Source: CAD feature listing. Evaluate the final solid. Frame: model axes, mm. A direction names the side the tool comes from. Coordinates: 2 decimals unless noted, no trailing zeros. Loops run counter-clockwise (first coordinate to the right, second up) from the corner with the lowest first, then second, coordinate; pieces in that order, holes last.
from build123d import *

# Parameters (mm, degrees)
SKETCH1_W           = 32
SKETCH1_H           = 32
BOSS_EXTRUDE1_DEPTH = 10
SKETCH2_R           = 11
CUT_EXTRUDE1_DEPTH  = 7
SKETCH3_R           = 2
SKETCH3_R_2         = 7.5
CUT_EXTRUDE2_DEPTH  = 11


with BuildPart() as part:
    # Sketch1 → Boss-Extrude1 (new body)
    with BuildSketch(Plane(origin=(0, 0, 0), x_dir=(1, 0, 0), z_dir=(0, 1, 0))):
        Rectangle(SKETCH1_W, SKETCH1_H)
    extrude(amount=BOSS_EXTRUDE1_DEPTH)

    # Sketch2 → Cut-Extrude1 (cut)
    with BuildSketch(Plane(origin=(0, 10, 0), x_dir=(1, 0, 0), z_dir=(0, 1, 0))):
        Circle(SKETCH2_R)
    extrude(amount=-CUT_EXTRUDE1_DEPTH, mode=Mode.SUBTRACT)

    # Sketch3 → Cut-Extrude2 (cut, through all)
    with BuildSketch(Plane(origin=(0, 10, 0), x_dir=(1, 0, 0), z_dir=(0, 1, 0))):
        with Locations((-12, 12)):
            Circle(SKETCH3_R)
        with Locations((12, 12)):
            Circle(SKETCH3_R)
        with Locations((12, -12)):
            Circle(SKETCH3_R)
        with Locations((-12, -12)):
            Circle(SKETCH3_R)
        Circle(SKETCH3_R_2)
    extrude(amount=-CUT_EXTRUDE2_DEPTH, mode=Mode.SUBTRACT)


solid = part.part
Q1. Section B-B, the plane y = 6. Return the cut outline in (x, z), plus the area to 3 significant figures.
Q2. Access query for faces 5 (the flat face through (16, 5, 0)), 6 (the cylindrical face through (-2.38, 6.55, 10.74)). Directions: +Z, -Z, +X, -X, +Y, -Y. A direction counts if a zero-diameter tool reaches every point of the face in a straight line with its end or side. Return the directions, or none.
Q3. Contact query for flat-ended pins moving along their axis: pin 1 Ø5 at (x, z) = (12, -12) entering from -Y; pin 2 Ø3.5 at (x, z) = (-12, -12) entering from +Y; pin 3 Ø17 at (x, z) = (0, 0) entering from +Y. Output: stop coordinate, or through.
Q4. Section C-C, the plane x = -12. Return the cut outline in (y, z), plus the area to 3 significant figures.
Q5. Line query: line 1 along Z through (x, y) = (12, 5.5); line 2 along X through (y, z) = (7, 0). Output: solid intervals per line, ascending.
Q6. Section D-D, the plane z = 0. Return the cut outline in (x, y), plus the area to 3 significant figures.
Q7. Section A-A, the plane z = -12. Return the cut outline in (x, y), plus the area to 3 significant figures.
Q8. Draft query along Z for faces 1 (the flat face through (7.2, 3, -2.6)), 2 (the flat face through (-16, 5, 0)), 3 (the flat face through (0, 5, -16)), 4 (the cylindrical face through (-12, 5, -14)). Return one class per face: +Z half, -Z half, draft (parallel to the pull), parting line (faces both ways), or undercut.
Derived:
1. outline: (-16, -16) - (16, -16) - (16, 16) - (-16, 16) - close; hole circle Ø4 at (-12, -12); hole circle Ø4 at (-12, 12); hole circle Ø22 at (0, 0); hole circle Ø4 at (12, -12); hole circle Ø4 at (12, 12)
1. area: 594 mm2
2. face 5: +Z, -Z, +X, +Y, -Y
2. face 6: +Y
3. pin 1: stops at y = 0
3. pin 2: passes through
3. pin 3: stops at y = 3
4. outline: (0, -16) - (10, -16) - (10, -14) - (0, -14) - close; (0, -10) - (10, -10) - (10, 10) - (0, 10) - close; (0, 14) - (10, 14) - (10, 16) - (0, 16) - close
4. area: 240 mm2
5. line 1: z = -16 to -14, -10 to 10, 14 to 16
5. line 2: x = -16 to -11, 11 to 16
6. outline: (-16, 0) - (-7.5, 0) - (-7.5, 3) - (-11, 3) - (-11, 10) - (-16, 10) - close; (7.5, 0) - (16, 0) - (16, 10) - (11, 10) - (11, 3) - (7.5, 3) - close
6. area: 121 mm2
7. outline: (-16, 0) - (-14, 0) - (-14, 10) - (-16, 10) - close; (-10, 0) - (10, 0) - (10, 10) - (-10, 10) - close; (14, 0) - (16, 0) - (16, 10) - (14, 10) - close
7. area: 240 mm2
8. face 1: undercut
8. face 2: draft
8. face 3: -Z half
8. face 4: undercut
